Source: CAD feature listing. Evaluate the final solid. Frame: model axes, mm. Round coordinates to 2 decimals unless told otherwise and drop trailing zeros. Write each loop counter-clockwise with the first axis right and the second up, starting at its lowest first coordinate (ties: lowest second). Pieces come first, ordered by that corner, then holes. Notation, with made-up numbers: M 86.5,73 L 120.5,73 A20 cw 120.5,87 Z; hole C 37.25,57 d7. An arc over 180 degrees is marked long. Put each result on its own line as item: value. Start each with the question number.
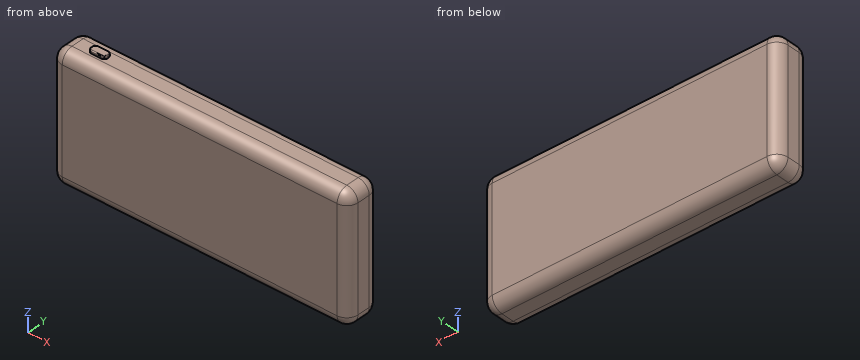
```python
from build123d import *
from OCP.BRepFilletAPI import BRepFilletAPI_MakeFillet

# Parameters (mm, degrees)
SKETCH1_W           = 160
SKETCH1_H           = 68
BOSS_EXTRUDE1_DEPTH = 19
FILLET1_R           = 6
SKETCH2_W           = 9
SKETCH2_H           = 4.5
BOSS_EXTRUDE2_DEPTH = 1.5
FILLET2_R1          = 2
FILLET2_R2          = 0.5


with BuildPart() as part:
    # Sketch1 → Boss-Extrude1 (new body)
    with BuildSketch(Plane(origin=(0, 0, 0), x_dir=(1, 0, 0), z_dir=(0, 1, 0))):
        Rectangle(SKETCH1_W, SKETCH1_H)
    extrude(amount=BOSS_EXTRUDE1_DEPTH)

    # Fillet1
    fillet1_edges = [part.edges().sort_by_distance(p)[0] for p in [
        (-80, 19, 0),
        (0, 19, 34),
        (80, 19, 0),
        (0, 0, 34),
        (-80, 0, 0),
        (0, 0, -34),
        (80, 0, 0),
        (80, 9.5, 34),
        (-80, 9.5, 34),
        (-80, 9.5, -34),
        (80, 9.5, -34),
        (0, 19, -34),
    ]]
    fillet(fillet1_edges, radius=FILLET1_R)

    # Sketch2 → Boss-Extrude2 (add)
    with BuildSketch(Plane.XY.offset(34)):
        with Locations((-62, 9.5)):
            Rectangle(SKETCH2_W, SKETCH2_H)
    extrude(amount=BOSS_EXTRUDE2_DEPTH)

    # Fillet2: one fillet with a radius per group of edges: ONE call of the kernel's fillet builder (fillet() takes one radius for all edges)
    fillet2_edges_1 = [part.edges().sort_by_distance(p)[0] for p in [
        (-57.5, 7.25, 34.75),
        (-57.5, 11.75, 34.75),
        (-66.5, 11.75, 34.75),
        (-66.5, 7.25, 34.75),
    ]]
    fillet2_edges_2 = [part.edges().sort_by_distance(p)[0] for p in [
        (-57.5, 9.5, 35.5),
        (-62, 11.75, 35.5),
        (-66.5, 9.5, 35.5),
        (-62, 7.25, 35.5),
    ]]
    fillet2 = BRepFilletAPI_MakeFillet(part.part.solid().wrapped)
    for e in fillet2_edges_1:
        fillet2.Add(FILLET2_R1, e.wrapped)
    for e in fillet2_edges_2:
        fillet2.Add(FILLET2_R2, e.wrapped)
    add(Compound.cast(fillet2.Shape()), mode=Mode.REPLACE)


solid = part.part
```
(1) Section query B-B (y = 3.75). Return loops of the section in (x, z).
(2) Contact query for flat-ended pins moving along their axis: P1, Ø5.5, axis at x = -6.5, y = 9, coming from the +Z side; P2, Ø0.5, axis at x = -62, z = 34.5, coming from the +Y side. Output: stop coordinate, or through.
(3) Ray query, line 1 along Z through (x, y) = (15.5, 10.75); line 2 along X through (y, z) = (1.25, -13); line 3 along Y through (x, z) = (-37, 29). Return the intervals inside material, ascending.
(4) Section query A-A (x = -8.5). Return loops of the section in (y, z), and give its area (3 significant figures).
Entries:
1. outline: M -79.56,-28 A5.56 ccw -74,-33.56 L 74,-33.56 A5.56 ccw 79.56,-28 L 79.56,28 A5.56 ccw 74,33.56 L -74,33.56 A5.56 ccw -79.56,28 Z
2. P1: z = 34
2. P2: y = 11.75
3. line 1: -34 to 34
3. line 2: -77.67 to 77.67
3. line 3: 0.08 to 18.92
4. outline: M 0,-28 A6 ccw 6,-34 L 13,-34 A6 ccw 19,-28 L 19,28 A6 ccw 13,34 L 6,34 A6 ccw 0,28 Z
4. area: 1,260 mm2
